from build123d import *

# Parameters (mm, degrees)
F0_W     = 400
F0_H     = 350
F1_DEPTH = 1600
F2_W     = 190
F2_H     = 340
F3_DEPTH = 350
F4_DEPTH = 500
F5_DEPTH = 10


# Not quite as in the source:
# - a feature names something its author has since deleted; it is built from what else it names


with BuildPart() as f1:
    # F0 (on Top) → F1 (new body)
    with BuildSketch(Plane.XY):
        with Locations((200, 175)):
            Rectangle(F0_W, F0_H)
    extrude(amount=F1_DEPTH)

    # F2 (on face) → F3 (cut)
    with BuildSketch(Plane.XZ):
        with Locations((295, 1420)):
            Rectangle(F2_W, F2_H)
        with Locations((105, 1420)):
            Rectangle(F2_W, F2_H)
        with Locations((105, 1060)):
            Rectangle(F2_W, F2_H)
        with Locations((295, 1060)):
            Rectangle(F2_W, F2_H)
        with Locations((295, 700)):
            Rectangle(F2_W, F2_H)
        with Locations((105, 700)):
            Rectangle(F2_W, F2_H)
    extrude(amount=-F3_DEPTH, mode=Mode.SUBTRACT)

    # F4 (cut): a face of the model
    f4_faces = [f1.faces().sort_by_distance(p)[0] for p in [
        (200, 175, 0),
    ]]
    extrude(f4_faces, amount=-F4_DEPTH, mode=Mode.SUBTRACT)

    # F5 (cut): a face of the model
    f5_faces = [f1.faces().sort_by_distance(p)[0] for p in [
        (200, 175, 500),
    ]]
    extrude(f5_faces, amount=-F5_DEPTH, mode=Mode.SUBTRACT)


solid = f1.part
CAD build for the part. Positions are in the model's coordinates, mm. A direction names the side the tool comes from. Coordinates: 2 decimals unless noted, no trailing zeros. Loops run counter-clockwise (first coordinate to the right, second up) from the corner with the lowest first, then second, coordinate; pieces in that order, holes last. Notation, with made-up numbers: (23.25, 42) - (29.25, 42) arc R26 cw to (29.25, 62) - close; hole circle Ø10 at (86, 13). An arc over 180 degrees is marked (long way). Write item = value, one per line. Start each with the question number.
Q1. Drill centre lines: L1, parallel to Z at x = 212, y = 156; L2, parallel to X at y = 220, z = 832. Where is each one in solid material? Low to high.
Q2. Cut at B-B, the plane x = 92. List the corners of the cut face in (y, z), then the cut area to 3 significant figures.
Q3. Which spindle directions (+Z, -Z, +X, -X, +Y, -Y) get a long thin tool onto all of the face, cutting with end or side? Do faces 4 (the flat face through (390, 173, 1058)), 5 (the flat face through (6, 350, 891)). Say none if no direction does.
Q4. Cut at C-C, the plane y = 294.5. List the corners of the cut face in (x, z).
Q5. Pull direction Z, two halves, no side cores. Call faces 1 (the flat face through (197, 177, 510)), 2 (the flat face through (197, 177, 1600)), 3 (the flat face through (10, 173, 1058)): pulls with the +Z half, pulls with the -Z half, needs draft (parallel to the pull), parting line crosses it, or undercut.
Q6. Cut at A-A, the plane z = 1394.5. List the corners of the cut face in (x, y), then the cut area to 3 significant figures.
Computed:
q1.L1 = 510 to 530, 870 to 890, 1230 to 1250, 1590 to 1600
q1.L2 = 0 to 10, 390 to 400
q2.outline = (0, 510) - (350, 510) - (350, 530) - (0, 530) - close; (0, 870) - (350, 870) - (350, 890) - (0, 890) - close; (0, 1230) - (350, 1230) - (350, 1250) - (0, 1250) - close; (0, 1590) - (350, 1590) - (350, 1600) - (0, 1600) - close
q2.area = 24,500 mm²
q3.face_4 = +Y, -Y
q3.face_5 = +Z, -Z, +X, -X, +Y
q4.outline = (0, 510) - (400, 510) - (400, 1600) - (0, 1600) - close; hole (10, 530) - (390, 530) - (390, 870) - (10, 870) - close; hole (10, 890) - (390, 890) - (390, 1230) - (10, 1230) - close; hole (10, 1250) - (390, 1250) - (390, 1590) - (10, 1590) - close
q5.face_1 = pulls with the -Z half
q5.face_2 = pulls with the +Z half
q5.face_3 = undercut
q6.outline = (0, 0) - (10, 0) - (10, 350) - (0, 350) - close; (390, 0) - (400, 0) - (400, 350) - (390, 350) - close
q6.area = 7,000 mm²
